Build history of the part. All positions in model axes, mm. A direction names the side the tool comes from. Give positions to 0.01 mm unless a question says otherwise; leave off trailing zeros. Order: outer loops, then holes, each group sorted by start corner. A loop starts at its lowest first (then second) coordinate and runs counter-clockwise, first axis right, second up. Notation, with made-up numbers: M -33.75,68.5 L 2.25,68.5 A10 cw 2.25,83.5 Z; hole C 76.5,83.5 d9. An arc over 180 degrees is marked long. One line per item, written item: value.
from build123d import *

# Parameters (mm, degrees)
CROQUIS1_W              = 37
CROQUIS1_H              = 44
SALIENTE_EXTRUIR1_DEPTH = 10.25
CROQUIS2_R              = 1.55
CORTAR_EXTRUIR1_DEPTH   = 10.25
CROQUIS3_W              = 1.5
CROQUIS3_H              = 44
CORTAR_EXTRUIR2_DEPTH   = 1
CROQUIS4_W              = 1.5
CROQUIS4_H              = 44
CORTAR_EXTRUIR3_DEPTH   = 1
CROQUIS5_R              = 1
CORTAR_EXTRUIR4_DEPTH   = 44
CROQUIS6_W              = 22
CROQUIS6_H              = 5
CORTAR_EXTRUIR5_DEPTH   = 5
REDONDEO1_R             = 10


with BuildPart() as part:
    # Croquis1 → Saliente-Extruir1 (new body)
    with BuildSketch(Plane(origin=(0, 0, 0), x_dir=(1, 0, 0), z_dir=(0, 1, 0))):
        with Locations((18.5, 22)):
            Rectangle(CROQUIS1_W, CROQUIS1_H)
    extrude(amount=SALIENTE_EXTRUIR1_DEPTH)

    # Croquis2 → Cortar-Extruir1 (cut)
    with BuildSketch(Plane(origin=(0, 10.25, 0), x_dir=(1, 0, 0), z_dir=(0, 1, 0))):
        with Locations(Location((19, 39, 0), (0, 0, 270))):
            Circle(CROQUIS2_R)
        with Locations(Location((19, 5.5, 0), (0, 0, 270))):
            Circle(CROQUIS2_R)
    extrude(amount=-CORTAR_EXTRUIR1_DEPTH, mode=Mode.SUBTRACT)

    # Croquis3 → Cortar-Extruir2 (cut)
    with BuildSketch(Plane(origin=(0, 10.25, 0), x_dir=(1, 0, 0), z_dir=(0, 1, 0))):
        with Locations((33.75, 22)):
            Rectangle(CROQUIS3_W, CROQUIS3_H)
    extrude(amount=-CORTAR_EXTRUIR2_DEPTH, mode=Mode.SUBTRACT)

    # Croquis4 → Cortar-Extruir3 (cut)
    with BuildSketch(Plane.XZ):
        with Locations((33.75, -22)):
            Rectangle(CROQUIS4_W, CROQUIS4_H)
    extrude(amount=-CORTAR_EXTRUIR3_DEPTH, mode=Mode.SUBTRACT)

    # Croquis5 → Cortar-Extruir4 (cut)
    with BuildSketch(Plane(origin=(0, 0, -44), x_dir=(-1, 0, 0), z_dir=(0, 0, -1))):
        with Locations((-33.75, 5.125)):
            Circle(CROQUIS5_R)
    extrude(amount=-CORTAR_EXTRUIR4_DEPTH, mode=Mode.SUBTRACT)

    # Croquis6 → Cortar-Extruir5 (cut)
    with BuildSketch(Plane.ZY):
        with Locations((-23, 6.75)):
            Rectangle(CROQUIS6_W, CROQUIS6_H)
    extrude(amount=-CORTAR_EXTRUIR5_DEPTH, mode=Mode.SUBTRACT)

    # Redondeo1
    # the kernel refuses this fillet: 10 mm, written as the material it takes off along each edge
    with BuildSketch(Plane(origin=(37, 0, 16.535945694), x_dir=(-1, 0, 0), z_dir=(0, 0, -1))) as redondeo1_piece_1:
        with BuildLine():
            CenterArc((10, 6.614378278), REDONDEO1_R, 180, 41.409622109)
            Line((0, 6.614378278), (-0.2, 6.614378278))
            Line((-0.2, 6.614378278), (-0.2, 0))
            Line((-0.2, 0), (0, -0.2))
            ThreePointArc((0, -0.2), (1.25, -0.2), (2.35, -0.132287566))
            Line((2.35, -0.132287566), (2.5, 0))
        make_face()
    extrude(amount=77.071891388, mode=Mode.SUBTRACT)
    with BuildSketch(Plane(origin=(37, 10.25, 16.535945694), x_dir=(0, -1, 0), z_dir=(0, 0, -1))) as redondeo1_piece_2:
        with BuildLine():
            CenterArc((6.614378278, 10), REDONDEO1_R, 228.590377891, 41.409622109)
            Line((0, 2.5), (-0.132287566, 2.35))
            ThreePointArc((-0.132287566, 2.35), (-0.2, 1.25), (-0.2, 0))
            Line((-0.2, 0), (0, -0.2))
            Line((0, -0.2), (6.614378278, -0.2))
            Line((6.614378278, -0.2), (6.614378278, 0))
        make_face()
    extrude(amount=77.071891388, mode=Mode.SUBTRACT)


solid = part.part
1) Saw through at D-D, the plane y = 8.75. Write the cut outline in (x, z), then the cut area to 3 significant figures.
Check values:
outline: M 0,-44 L 35.59,-44 L 35.59,0 L 0,0 L 0,-12 L 5,-12 L 5,-34 L 0,-34 Z; hole C 19,-39 d3.1; hole C 19,-5.5 d3.1
area: 1,440 mm^2
2) Drill centre lines: probe 1 along Z at (x, y) = (4, 8.5); probe 2 along X at (y, z) = (5.25, -40); probe 3 along X at (y, z) = (7.5, -5.5). Where is each one in solid material? Low to high. Write a range as from..to.
Check values:
probe 1: -44..-34, -12..0
probe 2: 0..17.82, 20.18..32.76, 34.74..36.87
probe 3: 0..17.45, 20.55..36.22
3) Mould opens along X. For faces 1 (the face through (5, 7, -23)), 2 (the face through (16, 10.25, -22)), 3 (the face through (36.047, 7.896, -21.692)), 4 (the face through (32.796, 5.425, -22.308)) say: released by +X, released by -X, zero draft, split by the parting line, or undercut.
Check values:
face 1: released by -X
face 2: zero draft
face 3: released by +X
face 4: undercut
4) Saw through at C-C, the plane z = -15. Write the cut outline in (x, y) (3 decimals).
Check values:
outline: M 0,0 L 33,0 L 33,1 L 34.5,1 L 34.5,0 A10 ccw 36.888,5.125 A10 ccw 34.5,10.25 L 34.5,9.25 L 33,9.25 L 33,10.25 L 0,10.25 L 0,9.25 L 5,9.25 L 5,4.25 L 0,4.25 Z; hole C 33.75,5.125 d2
5) Saw through at A-A, the plane z = -5.5. Write the cut outline in (x, y) (3 decimals), then the cut area to 3 significant figures.
Check values:
outline: M 0,0 L 17.45,0 L 17.45,10.25 L 0,10.25 Z; M 20.55,0 L 33,0 L 33,1 L 34.5,1 L 34.5,0 A10 ccw 36.888,5.125 A10 ccw 34.5,10.25 L 34.5,9.25 L 33,9.25 L 33,10.25 L 20.55,10.25 Z; hole C 33.75,5.125 d2
area: 331 mm^2
6) Tool access for faces 5 (the face through (2, 9.25, -23)), 6 (the face through (36.081, 2.427, -21.692)), 7 (the face through (34.5, 0.5, -22.3)), 8 (the face through (34, 9.25, -22)): list every direction of +Z, -Z, +X, -X, +Y, -Y with a clear straight run to the whole face (end or side of a thin tool).
Check values:
face 5: -X
face 6: +Z, -Z, +X, -Y
face 7: +Z, -Z, -Y
face 8: +Z, -Z, +Y
7) Pin check, flat tips, straight feed: pin 1 (2.5 mm diameter, centred on x = 19, z = -5.5, fed in from -Y); pin 2 (0.8 mm diameter, centred on y = 10, z = -26, fed in from +X); pin 3 (1.6 mm diameter, centred on x = 34, z = -29, fed in from -Y); pin 4 (2 mm diameter, centred on y = 2.5, z = -9, fed in from +X). Stop position of each tip, or through.
Check values:
pin 1: through
pin 2: x = 35.03
pin 3: y = 0
pin 4: x = 36.5
8) Saw through at B-B, the plane x = 19. Write the cut outline in (y, z), then the cut area to 3 significant figures.
Check values:
outline: M 0,-44 L 10.25,-44 L 10.25,-40.55 L 0,-40.55 Z; M 0,-37.45 L 10.25,-37.45 L 10.25,-7.05 L 0,-7.05 Z; M 0,-3.95 L 10.25,-3.95 L 10.25,0 L 0,0 Z
area: 387 mm^2
